Autodesk Inventor part; units mm, degrees
ref_plane "YZ Plane" through (0, 0, 0) normal (1, 0, 0) x (0, 1, 0)
ref_plane "XZ Plane" through (0, 0, 0) normal (0, 1, 0) x (-1, 0, 0)
ref_plane "XY Plane" through (0, 0, 0) normal (0, 0, 1) x (1, 0, 0)
sketch "草圖1" plane through (0, 0, 0) normal (0, 1, 0) x (-1, 0, 0)
  circle A0 centre (0, 0) radius 0.5
  dimension "d0" = 1
extrude "擠出1" add sketch "草圖1" along normal blind 10
sketch "草圖2" plane through (0, 10, 0) normal (0, 1, 0) x (1, 0, 0)
  circle A0 centre (0, 0) radius 1
  dimension "d3" = 2
extrude "擠出2" add sketch "草圖2" along normal blind 3
chamfer "倒角1" distance 1 distance2 3 1 edges at (-1, 13, 0) measured on face at (0.5848, 13, 0.397)
properties part number "Arrow"
Geometry check sheet. Reference: the model listing, model coordinates, mm. A direction names the side the tool comes from. Coordinates: 2 decimals unless noted, no trailing zeros. Order: outer loops, then holes, each group sorted by start corner. A loop starts at its lowest first (then second) coordinate and runs counter-clockwise, first axis right, second up. Notation, with made-up numbers: (-15, 81) - (3, 81) arc R28 ccw to (3, 112) - close; hole circle Ø6 at (6.5, 31). An arc over 180 degrees is marked (long way). Answer in a Markdown table with one row per item. Add a question column.
1. Gauge pin test, flat end, axial feed: pin 1 Ø1 at (y, z) = (5, 0) entering from -X. Record the tip position at first contact, or that the pin passes through.
2. Section check B-B (y = 12). Enter the section's corners in (x, z).
3. Section check A-A (y = 8). Enter the section's corners in (x, z).
4. Access from +Z, -Z, +X, -X, +Y, -Y to the whole of each face (thin tool, end or side, straight path). Record for faces 1 (the face through (0, 0, 0)), 2 (the face through (0.108, 4.93, 0.488)).
5. Material ranges on L1, parallel to Z at x = 0.05, y = 7.75; L2, parallel to X at y = 4, z = 0.3; L3, parallel to Y at x = 0.3, z = 0.3, recorded low to high. Write a range as [from, to].
Data:
| question | item | result |
|---|---|---|
| 1 | pin 1 | stops at x = -0.5 |
| 2 | outline | circle Ø0.67 at (0, 0) |
| 3 | outline | circle Ø1 at (0, 0) |
| 4 | face 1 | +Z, -Z, +X, -X, -Y |
| 4 | face 2 | -Y |
| 5 | L1 | z = [-0.5, 0.5] |
| 5 | L2 | x = [-0.4, 0.4] |
| 5 | L3 | y = [0, 11.73] |
